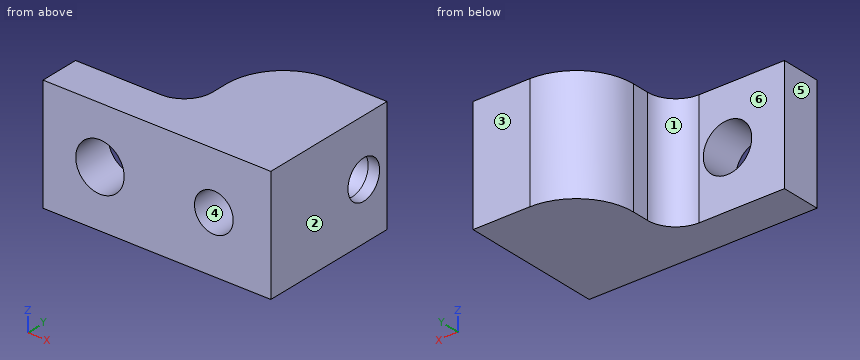
```python
from build123d import *

# Parameters (mm, degrees)
EXTRUDE_1_DEPTH     = 10
SKETCH_2_R          = 4.25
CUT_EXTRUDE_1_DEPTH = 8
SKETCH_4_R          = 3.4
FILLET_1_R          = 5
FILLET_2_R          = 10


with BuildPart() as part:
    # 草圖1 → 填料-伸長1 (new body, symmetric)
    with BuildSketch(Plane.XY):
        Polygon((20, 0), (20, 25), (0, 25), (0, 7), (-20, 7), (-20, 0), align=None)
    extrude(amount=EXTRUDE_1_DEPTH, both=True)

    # 草圖2 → 除料-伸長1 (cut, through all)
    with BuildSketch(Plane(origin=(0, 7, 0), x_dir=(1, 0, 0), z_dir=(0, 1, 0))):
        with Locations((-10, 0)):
            Circle(SKETCH_2_R)
    extrude(amount=-CUT_EXTRUDE_1_DEPTH, mode=Mode.SUBTRACT)

    # 除料-掃出1: sweep along a path in 草圖5
    with BuildLine(Plane(origin=(20, 0, 0), x_dir=(-1, 0, 0), z_dir=(0, 0, -1))) as sweep_1_path:
        Line((10, 0), (10, 12))
        ThreePointArc((10, 12), (7.656854249, 17.656854249), (2, 20))
        Line((2, 20), (0, 20))
    # 草圖4 → 除料-掃出1 (sweep, cut)
    with BuildSketch(Plane.XZ):
        with Locations((10, 0)):
            Circle(SKETCH_4_R)
    sweep(path=sweep_1_path.line, mode=Mode.SUBTRACT)

    # 圓角1
    fillet_1_edges = [part.edges().sort_by_distance(p)[0] for p in [
        (0, 7, 0),
    ]]
    fillet(fillet_1_edges, radius=FILLET_1_R)

    # 圓角2
    fillet_2_edges = [part.edges().sort_by_distance(p)[0] for p in [
        (0, 25, 0),
    ]]
    fillet(fillet_2_edges, radius=FILLET_2_R)


solid = part.part
```
CAD build for the part. Positions are in the model's coordinates, mm. Face numbers are marked on the shaded views. A direction names the side the tool comes from. Coordinates: 2 decimals unless noted, no trailing zeros. Loops run counter-clockwise (first coordinate to the right, second up) from the corner with the lowest first, then second, coordinate; pieces in that order, holes last. Notation, with made-up numbers: (39.5, 69.25) - (48.5, 69.25) arc R25 ccw to (48.5, 89.25) - close; hole circle Ø5 at (-17, -1). An arc over 180 degrees is marked (long way). Return JSON: item names as keys, results as strings.
1. Band-saw the part on B-B (x = -10). Give the cut face in (y, z), and give its area (3 significant figures).
Result:
{"outline": "(0, -10) - (7, -10) - (7, -4.25) - (0, -4.25) - close; (0, 4.25) - (7, 4.25) - (7, 10) - (0, 10) - close", "area": "80.5 mm2"}
2. Band-saw the part on C-C (z = -6). Give the cut face in (x, y), and give its area (3 significant figures).
Result:
{"outline": "(-20, 0) - (20, 0) - (20, 25) - (10, 25) arc R10 ccw to (0, 15) - (0, 12) arc R5 cw to (-5, 7) - (-20, 7) - close", "area": "624 mm2"}
3. Drop flat-ended pins along their axis: pin 1 (7.5 mm diameter, centred on x = -14.5, z = -5, fed in from +Y); pin 2 (1 mm diameter, centred on y = 19, z = -2, fed in from -X); pin 3 (0.9 mm diameter, centred on y = 13.5, z = 0.5, fed in from -X); pin 4 (7 mm diameter, centred on x = -10, z = 0, fed in from -Y). Give the stop position or say it passes through.
Result:
{"pin 1": "stops at y = 7", "pin 2": "stops at x = 0.63", "pin 3": "stops at x = 0", "pin 4": "passes through"}
4. Band-saw the part on D-D (y = 11.5). Give the cut face in (x, z), and give its area (3 significant figures).
Result:
{"outline": "(-0.03, -10) - (20, -10) - (20, 10) - (-0.03, 10) - close; hole circle Ø6.8 at (10, 0)", "area": "364 mm2"}
5. Probe L1, parallel to X at y = 2, z = 0; L2, parallel to Y at x = -11, z = 6; L3, parallel to Z at x = 19.15, y = 20. List the from-to ranges inside material, lowest first. Write a range as from..to.
Result:
{"L1": "x = -20..-14.25, -5.75..6.6, 13.4..20", "L2": "y = 0..7", "L3": "z = -10..-3.4, 3.4..10"}
6. Band-saw the part on A-A (z = 0). Give the cut face in (x, y), and give its area (3 significant figures).
Result:
{"outline": "(-20, 0) - (-14.25, 0) - (-14.25, 7) - (-20, 7) - close; (-5.75, 0) - (6.6, 0) - (6.6, 12) arc R11.4 cw to (18, 23.4) - (20, 23.4) - (20, 25) - (10, 25) arc R10 ccw to (0, 15) - (0, 12) arc R5 cw to (-5, 7) - (-5.75, 7) - close; (13.4, 0) - (20, 0) - (20, 16.6) - (18, 16.6) arc R4.6 ccw to (13.4, 12) - close", "area": "384 mm2"}
7. Mould opens along X. For the marked faces 1, 2, 3 and 4 say: released by +X, released by -X, zero draft, split by the parting line, or undercut.
Result:
{"face 1": "released by -X", "face 2": "released by +X", "face 3": "zero draft", "face 4": "undercut"}
8. 3-axis set-ups, long thin cutter, end or side, ignore diameter. For the marked faces 5 and 6: which of +Z, -Z, +X, -X, +Y, -Y reach the whole face in a straight line?
Result:
{"face 5": "+Z, -Z, -X, +Y, -Y", "face 6": "+Z, -Z, -X, +Y"}
